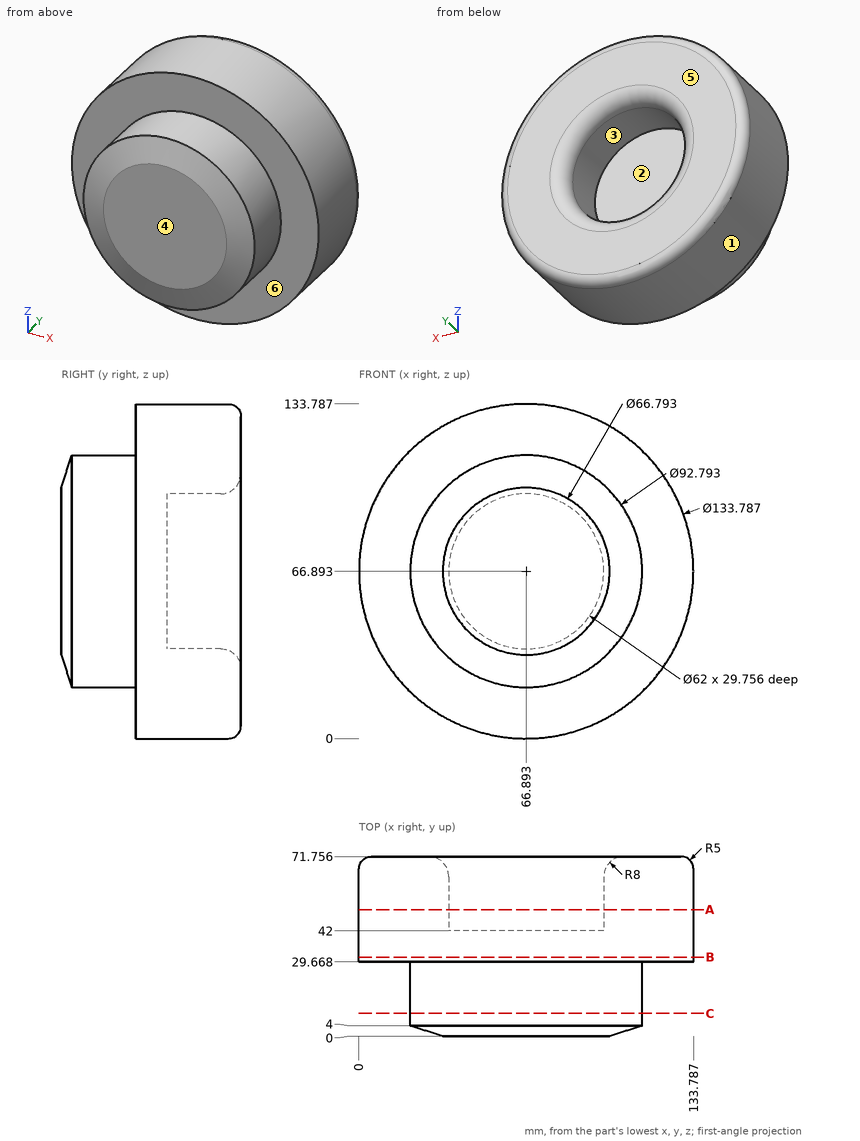
Print and shaded views of the part. All mm, measured from the part's lowest x, y and z. A direction names the side the tool comes from. Coordinates: 2 decimals unless noted, no trailing zeros. Order: outer loops, then holes, each group sorted by start corner. A loop starts at its lowest first (then second) coordinate and runs counter-clockwise, first axis right, second up.
(1) Tool access for the marked faces 5 and 6: list every direction of +Z, -Z, +X, -X, +Y, -Y with a clear straight run to the whole face (end or side of a thin tool).
Check sheet entries:
face 5: +Z, -Z, +X, -X, +Y
face 6: -Y
(2) Slice it at C-C, the plane y = 9. Write the cut outline in (x, z).
Check sheet entries:
outline: circle Ø92.79 at (66.89, 66.89)
(3) Slice it at A-A, the plane y = 50.5. Write the cut outline in (x, z).
Check sheet entries:
outline: circle Ø133.79 at (66.89, 66.89); hole circle Ø62 at (66.89, 66.89)
(4) Pin check, flat tips, straight feed: pin 1 Ø2 at (y, z) = (46, 80.5) entering from +X; pin 2 Ø2 at (x, y) = (32, 39.5) entering from -Z; pin 3 Ø18.5 at (x, z) = (80, 59) entering from +Y. Stop position of each tip, or through.
Check sheet entries:
pin 1: stops at x = 132.59
pin 2: stops at z = 9.22
pin 3: stops at y = 42
(5) Probe L1, parallel to Y at x = 39, z = 107 (1 decimal); L2, parallel to X at y = 45.5, z = 39.5 (1 decimal); L3, parallel to X at y = 63, z = 80.5. List the from-to ranges inside material, lowest first.
Check sheet entries:
L1: y = 29.7 to 71.8
L2: x = 5.9 to 52.4, 81.4 to 127.9
L3: x = 1.4 to 39.04, 94.75 to 132.39
(6) Slice it at B-B, the plane y = 31.5. Write the cut outline in (x, z).
Check sheet entries:
outline: circle Ø133.79 at (66.89, 66.89)
(7) Pull direction X, two halves, no side cores. Call the marked faces 1, 2, 3 and 4: pulls with the +X half, pulls with the -X half, needs draft (parallel to the pull), parting line crosses it, or undercut.
Check sheet entries:
face 1: parting line crosses it
face 2: undercut
face 3: undercut
face 4: needs draft
